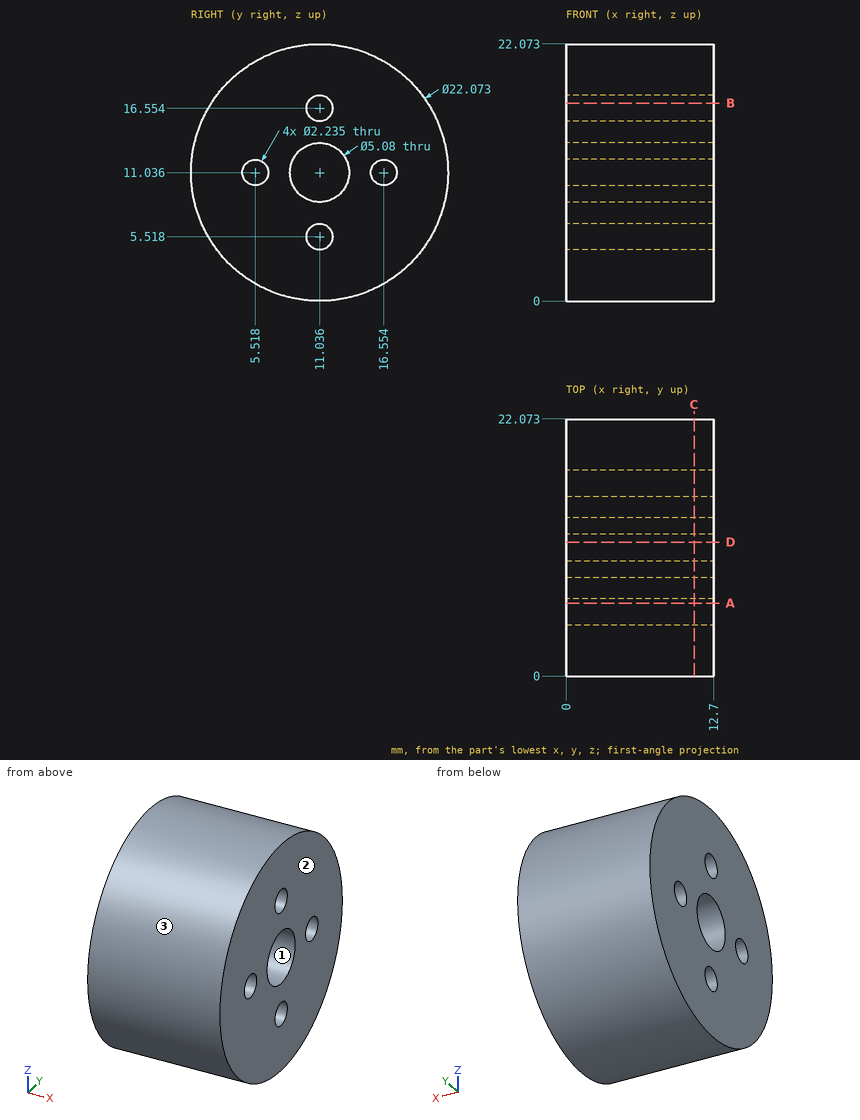
Verification items for this drawing (mm, ordinates from the low corner). Coordinates: 2 decimals unless noted, no trailing zeros. Write each loop counter-clockwise with the first axis right and the second up, starting at its lowest first coordinate (ties: lowest second). Pieces come first, ordered by that corner, then holes. Notation, with made-up numbers: (13, 26) -> (49, 26) arc R21 ccw to (49, 30) -> close; hole circle Ø9 at (-19.5, 53). An arc over 180 degrees is marked (long way). Use CSV: the item, a comma, the result in double quotes. Start each with the question number.
Item 1: Depth check by flat-ended pin: pin 1 Ø5 at (x, y) = (9, 7) entering from -Z; pin 2 Ø5 at (x, z) = (4, 4) entering from +Y. Enter the tip coordinate at first touch or a pass-through.
Item 2: Cross-section at A-A, the plane y = 6.25. Record the cut outline in (x, z).
Item 3: Cross-section at D-D, the plane y = 11.5. Record the cut outline in (x, z) (1 decimal), plus the area to 3 significant figures.
Item 4: Cross-section at C-C, the plane x = 11. Record the cut outline in (y, z) (1 decimal), plus the area to 3 significant figures.
Item 5: Cross-section at B-B, the plane z = 17. Record the cut outline in (x, y), plus the area to 3 significant figures.
Item 6: Mould release check, pull along Z, two halves, no side actions. Record for the marked faces 1, 2 and 3: released by +Z, released by -Z, zero draft, split by the parting line, or undercut.
Item 7: Thickness scan on line 1 (Z direction, x = 4, y = 11) (1 decimal); line 2 (Y direction, x = 2, z = 11.5) (1 decimal); line 3 (Y direction, x = 1.5, z = 12.25) (1 decimal). Record the ranges inside material, lowest first.
Answers:
1,pin 1,"z = 0.11"
1,pin 2,"y = 21.1"
2,outline,"(0, 1.09) -> (12.7, 1.09) -> (12.7, 10.19) -> (0, 10.19) -> close; (0, 11.88) -> (12.7, 11.88) -> (12.7, 20.98) -> (0, 20.98) -> close"
3,outline,"(0, 0) -> (12.7, 0) -> (12.7, 4.5) -> (0, 4.5) -> close; (0, 6.5) -> (12.7, 6.5) -> (12.7, 8.5) -> (0, 8.5) -> close; (0, 13.5) -> (12.7, 13.5) -> (12.7, 15.5) -> (0, 15.5) -> close; (0, 17.6) -> (12.7, 17.6) -> (12.7, 22.1) -> (0, 22.1) -> close"
3,area,"165 mm^2"
4,outline,"circle Ø22.1 at (11, 11); hole circle Ø2.2 at (5.5, 11); hole circle Ø5.1 at (11, 11); hole circle Ø2.2 at (11, 5.5); hole circle Ø2.2 at (11, 16.6); hole circle Ø2.2 at (16.6, 11)"
4,area,"347 mm^2"
5,outline,"(0, 1.75) -> (12.7, 1.75) -> (12.7, 10.01) -> (0, 10.01) -> close; (0, 12.06) -> (12.7, 12.06) -> (12.7, 20.32) -> (0, 20.32) -> close"
5,area,"210 mm^2"
6,face 1,"undercut"
6,face 2,"zero draft"
6,face 3,"split by the parting line"
7,line 1,"0 to 4.4, 6.6 to 8.5, 13.6 to 15.4, 17.7 to 22.1"
7,line 2,"0 to 4.5, 6.5 to 8.5, 13.5 to 15.5, 17.6 to 22.1"
7,line 3,"0.1 to 8.8, 13.3 to 22"
